The drawing under review shows one solid part. Ordinate dimensions are in mm from its lowest x, y, z. Coordinates: 2 decimals unless noted, no trailing zeros. Write each loop counter-clockwise with the first axis right and the second up, starting at its lowest first coordinate (ties: lowest second). Pieces come first, ordered by that corner, then holes. Notation, with made-up numbers: (89.25, 15) -> (143.25, 15) arc R17 ccw to (143.25, 29) -> close; hole circle Ø3 at (39, 50). An arc over 180 degrees is marked (long way). One line per item, written item: value. Start each with the question number.
1) Add section D-D (z = 20). State the section outline as (x, y) points.
2) For probe 1 along X at (y, z) = (5.5, 37); probe 2 along X at (y, z) = (10.75, 29); probe 3 along Y at (x, z) = (39, 19), list the stretches that pass through material, from the lowest coordinate up. Write a range as from..to.
3) Add section A-A (x = 38.1). State the section outline as (y, z) points.
4) Add section C-C (y = 6.25). State the section outline as (x, z) points.
5) For pin 1 Ø3 at (y, z) = (7, 18) entering from -X; pin 2 Ø1.3 at (y, z) = (12, 10.5) entering from +X; pin 3 Ø1.5 at (x, y) = (57, 4) entering from +Z, all flat-tipped, find the tip position at first contact; note any pin that passes through.
6) Add section B-B (z = 29). State the section outline as (x, y) points.
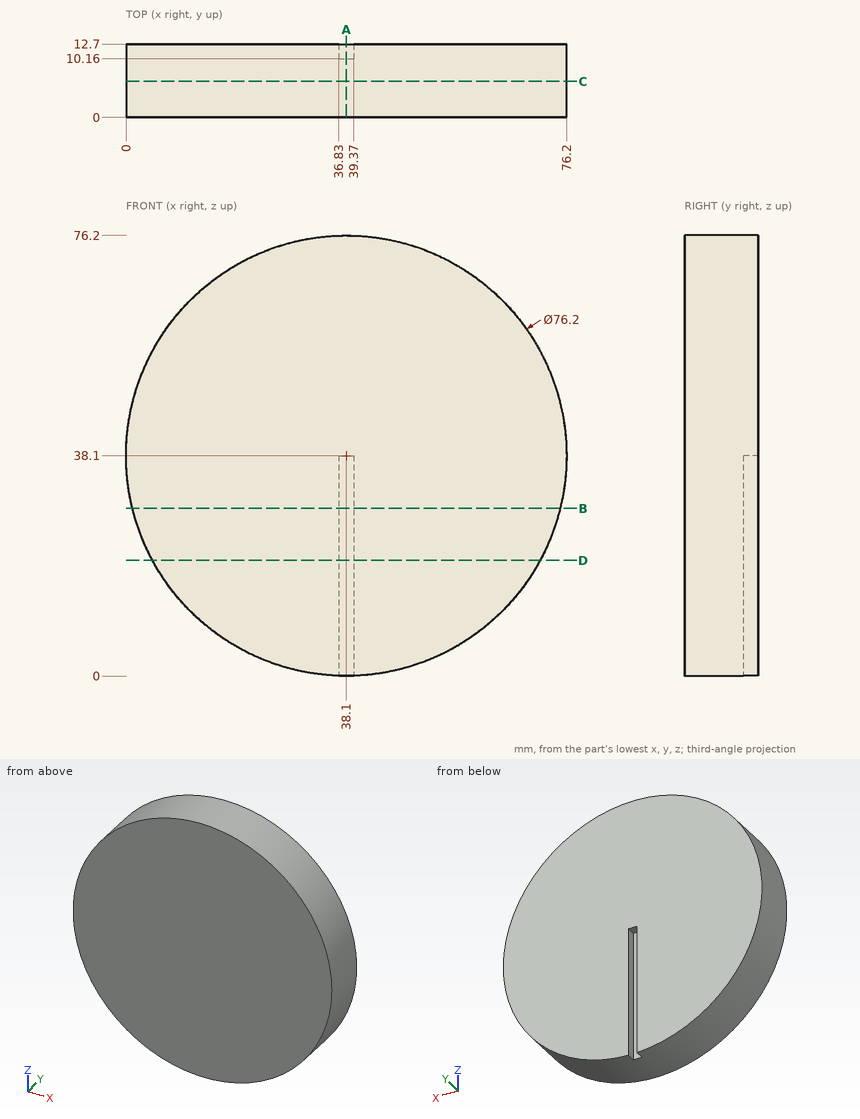
Numbers:
1. outline: (4.57, 0) -> (71.63, 0) -> (71.63, 12.7) -> (39.37, 12.7) -> (39.37, 10.16) -> (36.83, 10.16) -> (36.83, 12.7) -> (4.57, 12.7) -> close
2. probe 1: 0.02..76.18
2. probe 2: 1.1..36.83, 39.37..75.1
2. probe 3: 0..10.16
3. outline: (0, 0) -> (10.16, 0) -> (10.16, 38.1) -> (12.7, 38.1) -> (12.7, 76.2) -> (0, 76.2) -> close
4. outline: circle Ø76.2 at (38.1, 38.1)
5. pin 1: x = 4.85
5. pin 2: x = 65.03
5. pin 3: z = 71.6
6. outline: (1.1, 0) -> (75.1, 0) -> (75.1, 12.7) -> (39.37, 12.7) -> (39.37, 10.16) -> (36.83, 10.16) -> (36.83, 12.7) -> (1.1, 12.7) -> close
